Read the model definition and answer for the solid it produces. Units are mm, in the model's axes. A direction names the side the tool comes from. Round coordinates to 2 decimals unless told otherwise and drop trailing zeros. Loops run counter-clockwise (first coordinate to the right, second up) from the corner with the lowest first, then second, coordinate; pieces in that order, holes last. Notation, with made-up numbers: (82, 52.5) - (105, 52.5) arc R14 ccw to (105, 77.5) - close; hole circle Ø1 at (63.25, 38). An arc over 180 degrees is marked (long way). Use CSV: the item, a comma, the result in double quotes. Start each with the question number.
1. A tool of negligible diameter and unlimited length cuts with its end or side. For faces 1 (the flat face through (-15, 0, 11)), 2 (the flat face through (15, 0, 11)), 3 (the flat face through (0, -12, 6)), from which of +Z, -Z, +X, -X, +Y, -Y can it reach the whole face along a straight path? Write none if from no direction.
2. Consider line 1 along X through (y, z) = (11.75, 12); line 2 along Z through (x, y) = (-21.5, -27.85); line 3 along X through (y, z) = (-26, 7.75). Determine where each line is inside the solid, lowest interval first.
3. Find section C-C (y = -16). Give the vertices of the cut face in (x, z) (3 decimals), and give its area (3 significant figures).
4. Find section B-B (z = 3). State how many separate pieces and enclosed holes the cut face has, and give its area (4 significant figures).
5. Given pin 1 Ø3 at (x, z) = (21.5, 9) entering from +Y; pin 2 Ø3.5 at (x, y) = (-3, -24.25) entering from -Z; pin 3 Ø1.5 at (x, z) = (-9.5, 10.5) entering from -Y, each flat-ended and moving along its own axis, determine where each tip first touches the part or whether it passes through.
6. Determine the mould class of faces 4 (the cylindrical face through (-9.7, 14.1, 2.1)), 5 (the flat face through (0, 10, 0)), 6 (the flat face through (0, -6.75, 3)) for opening direction Z: +Z half, -Z half, draft (parallel to the pull), parting line (faces both ways), or undercut.
7. Find section A-A (x = -21.5). Give the vertices of the cut face in (y, z), and give its area (3 significant figures).
from build123d import *

# Parameters (mm, degrees)
F0_W      = 30
F0_H      = 30
F15_DEPTH = 18
F1_D      = 8
F1_DEPTH  = 6.5
F1_TIP    = 2.4034424761
F17_W     = 30
F17_H     = 2.5
F18_DEPTH = 6
F19_D     = 3
F19_DEPTH = 10
F19_TIP   = 0.9012909285
F2_R      = 1.475
F3_DEPTH  = 3.5
F20_W     = 23
F20_H     = 16
F21_DEPTH = 11.5
F22_R     = 3
F5_DEPTH  = 6
F22_R_2   = 1.5
F6_DEPTH  = 11.5
F7_R      = 1.55
F23_DEPTH = 16
F8_R      = 1.5
F9_DEPTH  = 8
F10_DEPTH = 6
F11_R     = 1.5
F12_DEPTH = 6


# Not quite as in the source:
# - a feature names something its author has since deleted; it is built from what else it names


with BuildPart() as f15:
    # F0 (on Top) → F15 (new body)
    with BuildSketch(Plane.XY):
        Rectangle(F0_W, F0_H)
    extrude(amount=F15_DEPTH)

    # F1
    with Locations(Plane(origin=(0, 15, 0), x_dir=(-1, 0, 0), z_dir=(0, 1, 0))):
        with Locations((-9, 12), (9, 12)):
            Hole(F1_D / 2, depth=F1_DEPTH)
            with Locations((0, 0, -(F1_DEPTH + F1_TIP / 2))):  # 118° drill point
                Cone(0, F1_D / 2, F1_TIP, mode=Mode.SUBTRACT)

    # F17 (on face) → F18 (cut)
    with BuildSketch(Plane(origin=(0, 0, 0), x_dir=(1, 0, 0), z_dir=(0, 0, -1))):
        with Locations((0, 12)):
            Rectangle(F17_W, F17_H)
        with Locations((0, 8)):
            Rectangle(F17_W, F17_H)
        with Locations((0, 4)):
            Rectangle(F17_W, F17_H)
        Rectangle(F17_W, F17_H)
        with Locations((0, -4)):
            Rectangle(F17_W, F17_H)
        with Locations((0, -8)):
            Rectangle(F17_W, F17_H)
        with Locations((0, -12)):
            Rectangle(F17_W, F17_H)
    extrude(amount=-F18_DEPTH, mode=Mode.SUBTRACT)

    # F19
    with Locations(Plane(origin=(0, 15, 0), x_dir=(-1, 0, 0), z_dir=(0, 1, 0))):
        with Locations((8.5, 3), (-8.5, 3), (0, 15)):
            Hole(F19_D / 2, depth=F19_DEPTH)
            with Locations((0, 0, -(F19_DEPTH + F19_TIP / 2))):  # 118° drill point
                Cone(0, F19_D / 2, F19_TIP, mode=Mode.SUBTRACT)

    # F2 (on face) → F3 (join)
    with BuildSketch(Plane.XZ.offset(15)):
        with Locations((-9, 12)):
            Circle(F2_R)
        with Locations((9, 12)):
            Circle(F2_R)
    extrude(amount=F3_DEPTH)

    # F20 (on offset) → F21 (join)
    with BuildSketch(Plane.XZ.offset(18.5)):
        with Locations((-12.5, 12)):
            Rectangle(F20_W, F20_H)
        with Locations((12.5, 12)):
            Rectangle(F20_W, F20_H)
    extrude(amount=F21_DEPTH)

    # F22 (on face) → F5 (cut)
    with BuildSketch(Plane.XZ.offset(30)):
        with Locations((-9, 12)):
            Circle(F22_R)
        with Locations((9, 12)):
            Circle(F22_R)
    extrude(amount=-F5_DEPTH, mode=Mode.SUBTRACT)

    # F22 (on face) → F6 (cut, through all)
    with BuildSketch(Plane.XZ.offset(30)):
        with Locations((-21.5, 12)):
            Circle(F22_R_2)
        with Locations((21.5, 12)):
            Circle(F22_R_2)
    extrude(amount=-F6_DEPTH, mode=Mode.SUBTRACT)

    # F7 (on face) → F23 (cut, through all)
    with BuildSketch(Plane.XY.offset(20)):
        with BuildLine():
            Line((-24, -26.75), (-18.4047375097, -26.75))
            ThreePointArc((-18.4047375097, -26.75), (-12.5, -26), (-18.4047375097, -25.25))
            Line((-18.4047375097, -25.25), (-24, -25.25))
            Line((-24, -25.25), (-24, -26.75))
        make_face()
        with Locations((-3, -24.25)):
            Circle(F7_R)
        with Locations((3, -24.25)):
            Circle(F7_R)
        with BuildLine():
            Line((18.4047375097, -26.75), (24, -26.75))
            Line((24, -26.75), (24, -25.25))
            Line((24, -25.25), (18.4047375097, -25.25))
            ThreePointArc((18.4047375097, -25.25), (12.5, -26), (18.4047375097, -26.75))
        make_face()
    extrude(amount=-F23_DEPTH, mode=Mode.SUBTRACT)

    # F8 (on face) → F9 (cut)
    with BuildSketch(Plane.XY.offset(18)):
        with Locations((0, -5)):
            Circle(F8_R)
        with Locations((4.5, 5)):
            Circle(F8_R)
        with Locations((-4.5, 5)):
            Circle(F8_R)
    extrude(amount=-F9_DEPTH, mode=Mode.SUBTRACT)

    # F22 (on face) → F10 (cut)
    with BuildSketch(Plane.XZ.offset(30)):
        with Locations((-9, 12)):
            Circle(F22_R)
    extrude(amount=-F10_DEPTH, mode=Mode.SUBTRACT)

    # F13: F12b, F12 across plane


with BuildPart() as f12:
    # F11 (on face) → F12 (new body)
    with BuildSketch(Plane.YZ.offset(15)):
        with Locations((-12, 12)):
            Circle(F11_R)
    extrude(amount=-F12_DEPTH)


with BuildPart() as f12b:
    # F11 (on face) → F12, piece 2 (new body)
    with BuildSketch(Plane.YZ.offset(15)):
        with Locations((-4, 12)):
            Circle(F11_R)
    extrude(amount=-F12_DEPTH)


with BuildPart() as f15_1:
    add(f15.part)
    add(f12b.part.mirror(Plane.YZ), mode=Mode.SUBTRACT)
    add(f12.part.mirror(Plane.YZ), mode=Mode.SUBTRACT)

    # F14: cut F12, F12b
    add(f12.part, mode=Mode.SUBTRACT)
    add(f12b.part, mode=Mode.SUBTRACT)


solid = f15_1.part
Filled sheet:
1,face 1,"+Z, -Z, -X, +Y"
1,face 2,"+Z, -Z, +X, +Y"
1,face 3,"-Z, +X, -X"
2,line 1,"x = -15 to -13, -5 to 5, 13 to 15"
2,line 2,"z = 4 to 10.5, 13.5 to 20"
2,line 3,"x = -12.5 to -1, 1 to 12.5"
3,outline,"circle Ø2.95 at (-9, 12); circle Ø2.95 at (9, 12)"
3,area,"13.7 mm²"
4,separate pieces,"14"
4,enclosed holes,"0"
4,area,"346.5 mm²"
5,pin 1,"stops at y = -18.5"
5,pin 2,"stops at z = 4"
5,pin 3,"stops at y = -24"
6,face 4,"undercut"
6,face 5,"-Z half"
6,face 6,"draft"
7,outline,"(-30, 4) - (-26.75, 4) - (-26.75, 10.5) - (-30, 10.5) - close; (-30, 13.5) - (-26.75, 13.5) - (-26.75, 20) - (-30, 20) - close; (-25.25, 4) - (-18.5, 4) - (-18.5, 10.5) - (-25.25, 10.5) - close; (-25.25, 13.5) - (-18.5, 13.5) - (-18.5, 20) - (-25.25, 20) - close"
7,area,"130 mm²"
